The listing builds one solid part. Answer for the finished solid, in the listing's coordinates (mm). A direction names the side the tool comes from. Coordinates: 2 decimals unless noted, no trailing zeros. Write each loop counter-clockwise with the first axis right and the second up, starting at its lowest first coordinate (ties: lowest second). Pieces come first, ordered by that corner, then holes. Notation, with made-up numbers: M 23.25,-0.75 L 30.25,-0.75 A10 cw 30.25,3.25 Z; hole C 88,30 d1. An arc over 180 degrees is marked long. Put each result on its own line as item: value. Start each with the question number.
```python
from build123d import *

# Parameters (mm, degrees)
BOSS_EXTRUDE1_DEPTH = 10
SKETCH3_R           = 3
BOSS_EXTRUDE2_DEPTH = 7
SKETCH4_R           = 2.75
CUT_EXTRUDE1_DEPTH  = 64.215786076
SKETCH5_W           = 5
SKETCH5_H           = 40.7
CUT_EXTRUDE2_DEPTH  = 7
SKETCH6_R           = 4.5
CUT_EXTRUDE3_DEPTH  = 1.6


with BuildPart() as part:
    # Sketch2 → Boss-Extrude1 (new body)
    with BuildSketch(Plane.XY):
        Polygon((-24.382192178, 22.640051942), (-54.382192178, 4.940051942), (-54.382192178, -10.059948058), (25.617807822, -10.059948058), (25.617807822, 4.940051942), (-4.382192178, 22.640051942), (-4.382192178, 30.640051942), (-24.382192178, 30.640051942), align=None)
    extrude(amount=BOSS_EXTRUDE1_DEPTH)

    # Sketch3 → Boss-Extrude2 (add)
    with BuildSketch(Plane.XY.offset(10)):
        with Locations((-18.382192178, 26.640051942)):
            Circle(SKETCH3_R)
    boss_extrude2 = extrude(amount=BOSS_EXTRUDE2_DEPTH)

    # Mirror1: Boss-Extrude2 across plane
    add(boss_extrude2.mirror(Plane.ZY.offset(14.382192178)))

    # Sketch4 → Cut-Extrude1 (cut, through all)
    with BuildSketch(Plane.XY.offset(10)):
        with Locations((-37.952192178, -3.959948058)):
            Circle(SKETCH4_R)
    cut_extrude1 = extrude(amount=-CUT_EXTRUDE1_DEPTH, mode=Mode.SUBTRACT)

    # Mirror2: Cut-Extrude1 across plane
    add(cut_extrude1.mirror(Plane.ZY.offset(14.382192178)), mode=Mode.SUBTRACT)

    # Sketch5 → Cut-Extrude2 (cut)
    with BuildSketch(Plane.XY.offset(10)):
        with Locations((-14.382192178, 10.290051942)):
            Rectangle(SKETCH5_W, SKETCH5_H)
    extrude(amount=CUT_EXTRUDE2_DEPTH, mode=Mode.SUBTRACT)

    # Sketch6 → Cut-Extrude3 (cut)
    with BuildSketch(Plane.XY.offset(10)):
        with Locations((-37.952192178, -3.959948058)):
            Circle(SKETCH6_R)
        with Locations((9.187807822, -3.959948058)):
            Circle(SKETCH6_R)
    extrude(amount=-CUT_EXTRUDE3_DEPTH, mode=Mode.SUBTRACT)


solid = part.part
```
1) Given pin 1 Ø4.5 at (x, y) = (-38, -5.5) entering from +Z; pin 2 Ø8 at (x, y) = (-27.5, 22.5) entering from +Z; pin 3 Ø2.5 at (y, z) = (27.5, 13) entering from +X, each flat-ended and moving along its own axis, determine where each tip first touches the part or whether it passes through.
2) Determine the mould class of faces 6 (the face through (7, -6, 8.4)), 7 (the face through (-15, 6, 0)), 8 (the face through (-14, 30.64, 5)) for opening direction Y: +Y half, -Y half, draft (parallel to the pull), parting line (faces both ways), or undercut.
3) For faces 1 (the face through (-24.382, 27, 5)), 2 (the face through (-4.382, 27, 5)), 3 (the face through (-15, -10.06, 5)), 4 (the face through (-16.882, 27, 13)), 5 (the face through (-38, -7, 8.4)), determine the directions among +Z, -Z, +X, -X, +Y, -Y from which every point of the face is accessible in a straight line to the end or side of a thin tool.
4) Straight lines are drawn through the part: probe 1 along Z at (x, y) = (-10, 3.5); probe 2 along X at (y, z) = (-2, 8.5); probe 3 along X at (y, z) = (28, 11.75). For each, find the intervals that lie inside material, in ascending order.
5) A cutting plane is placed at D-D on x = -18. Write down the section's boundary in (y, z).
6) A cutting plane is placed at C-C on y = -3. Write down the section's boundary in (x, z).
7) A cutting plane is placed at A-A on x = -38.5. Write down the section's boundary in (y, z).
8) A cutting plane is placed at B-B on z = 12. Write down the section's boundary in (x, y), then the cut area to 3 significant figures.
Answers follow:
1. pin 1: stops at z = 8.4
1. pin 2: stops at z = 10
1. pin 3: stops at x = -7.38
2. face 6: undercut
2. face 7: draft
2. face 8: +Y half
3. face 1: +Z, -Z, -X, +Y
3. face 2: +Z, -Z, +X, +Y
3. face 3: +Z, -Z, +X, -X, -Y
3. face 4: +Z, +Y, -Y
3. face 5: +Z
4. probe 1: z = 0 to 10
4. probe 2: x = -54.38 to -42, -33.9 to 5.14, 13.24 to 25.62
4. probe 3: x = -21.06 to -16.88, -11.88 to -7.71
5. outline: M -10.06,0 L 30.64,0 L 30.64,10 L 29.62,10 L 29.62,17 L 23.66,17 L 23.66,10 L -10.06,10 Z
6. outline: M -54.38,0 L -40.53,0 L -40.53,8.4 L -42.35,8.4 L -42.35,10 L -54.38,10 Z; M -35.38,0 L 6.61,0 L 6.61,8.4 L 4.79,8.4 L 4.79,10 L -33.56,10 L -33.56,8.4 L -35.38,8.4 Z; M 11.76,0 L 25.62,0 L 25.62,10 L 13.58,10 L 13.58,8.4 L 11.76,8.4 Z
7. outline: M -10.06,0 L -6.65,0 L -6.65,8.4 L -8.43,8.4 L -8.43,10 L -10.06,10 Z; M -1.27,0 L 14.31,0 L 14.31,10 L 0.51,10 L 0.51,8.4 L -1.27,8.4 Z
8. outline: M -16.88,24.04 L -16.88,29.24 A3 ccw long Z; M -11.88,24.04 A3 ccw long -11.88,29.24 Z
8. area: 45.5 mm²
